Verification items for the finished model (mm, model axes). Give positions to 0.01 mm unless a question says otherwise; leave off trailing zeros. Write each loop counter-clockwise with the first axis right and the second up, starting at its lowest first coordinate (ties: lowest second). Pieces come first, ordered by that corner, then holes. Notation, with made-up numbers: (86, 28.25) -> (133, 28.25) arc R35 ccw to (133, 60.25) -> close; hole circle Ø3 at (34, 21). An arc over 180 degrees is marked (long way). Answer as CSV lines item,"result". Start each with the question number.
1) Sectioned sample at A-A on z = -6. Record the cut outline in (x, y) (3 decimals).
2) Gauge pin test, flat end, axial feed: pin 1 Ø2 at (x, z) = (51.825, -6) entering from -Y. Record the tip position at first contact, or that the pin passes through.
3) Material ranges on L1, parallel to X at y = -1.45, z = -6 (3 decimals); L2, parallel to X at y = 2.25, z = 4.75, recorded low to high.
4) Sectioned sample at B-B on y = -1.2. Record the cut outline in (x, z) (3 decimals).
```python
from build123d import *

# Parameters (mm, degrees)
SKETCH1_W            = 110
SKETCH1_H            = 20
BOSS_EXTRUDE1_DEPTH  = 2.5
M3_CLEARANCE_HOLE1_D = 3.6


with BuildPart() as part:
    # Sketch1 → Boss-Extrude1 (new, symmetric)
    with BuildSketch(Plane(origin=(0, 0, 0), x_dir=(1, 0, 0), z_dir=(0, 1, 0))):
        Rectangle(SKETCH1_W, SKETCH1_H)
    extrude(amount=BOSS_EXTRUDE1_DEPTH, both=True)

    # M3 Clearance Hole1 (through all)
    with Locations(Plane(origin=(0, 2.5, 0), x_dir=(1, 0, 0), z_dir=(0, 1, 0))):
        with Locations((51.825, 6), (-51.825, -6), (51.825, -6), (-51.825, 6)):
            Hole(M3_CLEARANCE_HOLE1_D / 2)


solid = part.part
```
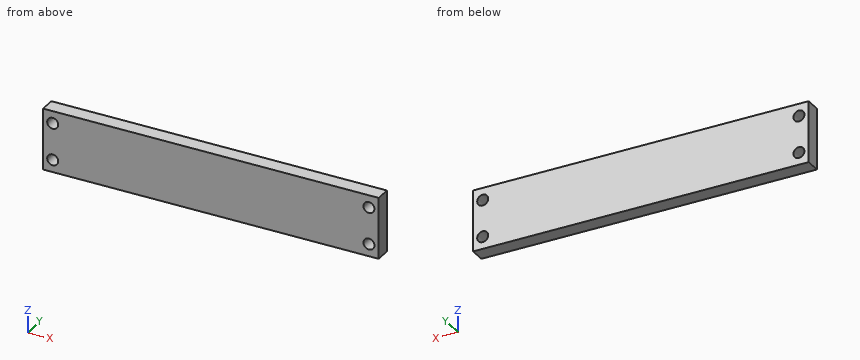
Ans:
1,outline,"(-55, -2.5) -> (-53.625, -2.5) -> (-53.625, 2.5) -> (-55, 2.5) -> close; (-50.025, -2.5) -> (50.025, -2.5) -> (50.025, 2.5) -> (-50.025, 2.5) -> close; (53.625, -2.5) -> (55, -2.5) -> (55, 2.5) -> (53.625, 2.5) -> close"
2,pin 1,"passes through"
3,L1,"x = -55 to -53.625, -50.025 to 50.025, 53.625 to 55"
3,L2,"x = -55 to -53.12, -50.53 to 50.53, 53.12 to 55"
4,outline,"(-55, -10) -> (55, -10) -> (55, 10) -> (-55, 10) -> close; hole circle Ø3.6 at (-51.825, -6); hole circle Ø3.6 at (-51.825, 6); hole circle Ø3.6 at (51.825, -6); hole circle Ø3.6 at (51.825, 6)"
